from build123d import *

# Parameters (mm, degrees)
BOSS_EXTRUDE1_DEPTH    = 1.5
SKETCH2_W              = 30
SKETCH2_H              = 40
BOSS_EXTRUDE2_DEPTH    = 1.5
CONVERT_SOLID1_START   = -20
CONVERT_SOLID1_DEPTH   = 40
CONVERT_SOLID1_2_DEPTH = 40
M3_CLEARANCE_HOLE1_D   = 3.2
CIRPATTERN1_COUNT      = 6
CUT_EXTRUDE1_DEPTH     = 46.650848842
FILLET1_R              = 3
CUT_EXTRUDE2_DEPTH     = 1.5


# Read off the part's stored shape, not the designer's step: Convert-Solid1
with BuildPart() as part:
    # Sketch1 → Boss-Extrude1 (new body)
    with BuildSketch(Plane(origin=(0, 0, 0), x_dir=(0, 0, -1), z_dir=(1, 0, 0))):
        with BuildLine():
            Line((-20, 0), (-20, -28))
            Line((-20, -28), (20, -28))
            Line((20, -28), (20, 0))
            ThreePointArc((20, 0), (0, 20), (-20, 0))
        make_face()
    extrude(amount=BOSS_EXTRUDE1_DEPTH)

    # Sketch2 → Boss-Extrude2 (add)
    with BuildSketch(Plane.XZ.offset(28)):
        with Locations((15, 0)):
            Rectangle(SKETCH2_W, SKETCH2_H)
    extrude(amount=-BOSS_EXTRUDE2_DEPTH)

    # Convert-Solid1 outline → Convert-Solid1 (cut)
    with BuildSketch(Plane.XY.offset(CONVERT_SOLID1_START)):
        with BuildLine():
            Line((0, -28), (2.262, -28))
            ThreePointArc((2.262, -28), (0.662524461, -27.337475539), (0, -25.738))
            Line((0, -25.738), (0, -28))
        make_face()
    extrude(amount=CONVERT_SOLID1_DEPTH, mode=Mode.SUBTRACT)

    # Convert-Solid1 2 outline → Convert-Solid1 2 (add)
    with BuildSketch(Plane.XY.offset(CONVERT_SOLID1_START)):
        with BuildLine():
            Line((1.5, -26.5), (2.262, -26.5))
            ThreePointArc((2.262, -26.5), (1.723184633, -26.276815367), (1.5, -25.738))
            Line((1.5, -25.738), (1.5, -26.5))
        make_face()
    extrude(amount=CONVERT_SOLID1_2_DEPTH)

    # M3 Clearance Hole1 (through all)
    with Locations(Plane.ZY):
        with Locations((-15.5, 0)):
            m3_clearance_hole1 = Hole(M3_CLEARANCE_HOLE1_D / 2)

    # CirPattern1: M3 Clearance Hole1 ×6 about axis
    cirpattern1_axis = Axis((0, 0, 0), (1, 0, 0))
    for i in range(1, CIRPATTERN1_COUNT):
        add(m3_clearance_hole1.rotate(cirpattern1_axis, i * 360 / CIRPATTERN1_COUNT), mode=Mode.SUBTRACT)

    # Sketch9 → Cut-Extrude1 (cut, through all)
    with BuildSketch(Plane.ZY):
        with BuildLine():
            Line((6.25, 7), (6.25, -7))
            ThreePointArc((6.25, -7), (0, -13.25), (-6.25, -7))
            Line((-6.25, -7), (-6.25, 7))
            ThreePointArc((-6.25, 7), (0, 13.25), (6.25, 7))
        make_face()
    extrude(amount=-CUT_EXTRUDE1_DEPTH, mode=Mode.SUBTRACT)

    # Fillet1
    fillet1_edges = [part.edges().sort_by_distance(p)[0] for p in [
        (30, -27.25, 20),
        (30, -27.25, -20),
    ]]
    fillet(fillet1_edges, radius=FILLET1_R)

    # Sketch10 → Cut-Extrude2 (cut)
    with BuildSketch(Plane(origin=(0, -28, 0), x_dir=(-1, 0, 0), z_dir=(0, -1, 0))):
        with BuildLine():
            Line((-9.5, -16.65), (-23.5, -16.65))
            ThreePointArc((-23.5, -16.65), (-25.6, -14.55), (-23.5, -12.45))
            Line((-23.5, -12.45), (-9.5, -12.45))
            ThreePointArc((-9.5, -12.45), (-7.4, -14.55), (-9.5, -16.65))
        make_face()
        with BuildLine():
            Line((-7.4, 7), (-7.4, -7))
            ThreePointArc((-7.4, -7), (-9.5, -9.1), (-11.6, -7))
            Line((-11.6, -7), (-11.6, 7))
            ThreePointArc((-11.6, 7), (-9.5, 9.1), (-7.4, 7))
        make_face()
        with BuildLine():
            Line((-21.4, 7), (-21.4, -7))
            ThreePointArc((-21.4, -7), (-23.5, -9.1), (-25.6, -7))
            Line((-25.6, -7), (-25.6, 7))
            ThreePointArc((-25.6, 7), (-23.5, 9.1), (-21.4, 7))
        make_face()
        with BuildLine():
            Line((-9.5, 16.65), (-23.5, 16.65))
            ThreePointArc((-23.5, 16.65), (-25.6, 14.55), (-23.5, 12.45))
            Line((-23.5, 12.45), (-9.5, 12.45))
            ThreePointArc((-9.5, 12.45), (-7.4, 14.55), (-9.5, 16.65))
        make_face()
    extrude(amount=-CUT_EXTRUDE2_DEPTH, mode=Mode.SUBTRACT)


solid = part.part
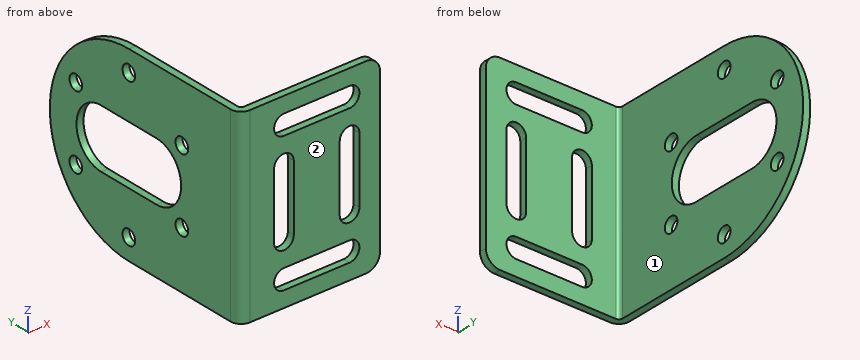
Design review of the part built by this model. Coordinates are the model's own, in mm. Face numbers are marked on the shaded views. A direction names the side the tool comes from. Coordinates: 2 decimals unless noted, no trailing zeros. Loops run counter-clockwise (first coordinate to the right, second up) from the corner with the lowest first, then second, coordinate; pieces in that order, holes last. Notation, with made-up numbers: (-35.75, -32) -> (-12.75, -32) arc R23 cw to (-12.75, 7) -> close; hole circle Ø5 at (30.25, 24.5). An arc over 180 degrees is marked (long way). Use a Markdown table: item, result. Add a question column.
Item 1: We need section B-B, the plane z = 0.5. Write out the cut boundary in (x, y), and give its area (3 significant figures).
Item 2: Clearance check with flat-ended pins moving along their axes: P1, Ø6, axis at y = 5.5, z = 8.5, coming from the +X side; P2, Ø1, axis at x = 14.5, z = 7.5, coming from the +Y side; P3, Ø0.8, axis at y = -27.5, z = 1, coming from the -X side. State where each tip first meets the part, or that it passes through.
Item 3: We need section D-D, the plane z = -15.5. Write out the cut boundary in (x, y), and give its area (3 significant figures).
Item 4: Wall thickness on L1, parallel to Y at x = 27.5, z = -17; L2, parallel to Y at x = 0.55, z = 7.75; L3, parallel to X at y = -9.5, z = -10: over which ranges is each line inside the solid? List them lowest first. Write a range as from..to.
Item 5: We need section C-C, the plane y = 1. Write out the cut boundary in (x, z), and give its area (3 significant figures).
Item 6: Machinability: for the marked faces 1 and 2, which of the approach directions +Z, -Z, +X, -X, +Y, -Y give a long, thin tool a straight path to every point of the face, cutting with its end or side? Answer none if there is none.
Item 7: We need section A-A, the plane x = 18.75. Write out the cut boundary in (y, z).
Numbers:
| question | item | result |
|---|---|---|
| 1 | outline | (0, -25.74) arc R2.26 ccw to (2.26, -28) -> (7.4, -28) -> (7.4, -26.5) -> (2.26, -26.5) arc R0.76 cw to (1.5, -25.74) -> (1.5, -13.23) -> (0, -13.23) -> close; (0, 13.23) -> (1.5, 13.23) -> (1.5, 19.99) -> (0, 19.99) -> close; (11.6, -28) -> (21.4, -28) -> (21.4, -26.5) -> (11.6, -26.5) -> close; (25.6, -28) -> (30, -28) -> (30, -26.5) -> (25.6, -26.5) -> close |
| 1 | area | 61.5 mm^2 |
| 2 | P1 | stops at x = 1.5 |
| 2 | P2 | stops at y = -26.5 |
| 2 | P3 | stops at x = 0.46 |
| 3 | outline | (0, -25.74) arc R2.26 ccw to (2.26, -28) -> (7.63, -28) -> (7.63, -26.5) -> (2.26, -26.5) arc R0.76 cw to (1.5, -25.74) -> (1.5, -1.6) -> (0, -1.6) -> close; (0, 1.6) -> (1.5, 1.6) -> (1.5, 12.64) -> (0, 12.64) -> close; (25.37, -28) -> (30, -28) -> (30, -26.5) -> (25.37, -26.5) -> close |
| 3 | area | 71.3 mm^2 |
| 4 | L1 | y = -28..-26.5 |
| 4 | L2 | y = -27.22..-15.02, -11.82..11.82, 15.02..18.44 |
| 4 | L3 | x = 0..1.5 |
| 5 | outline | (0, -19.97) -> (1.5, -19.97) -> (1.5, -16.75) -> (0, -16.75) -> close; (0, -14.25) -> (1.5, -14.25) -> (1.5, -6.25) -> (0, -6.25) -> close; (0, 6.25) -> (1.5, 6.25) -> (1.5, 14.25) -> (0, 14.25) -> close; (0, 16.75) -> (1.5, 16.75) -> (1.5, 19.97) -> (0, 19.97) -> close |
| 5 | area | 33.7 mm^2 |
| 6 | face 1 | +Z, -Z, +X, +Y |
| 6 | face 2 | +Z, -Z, +X, -X, -Y |
| 7 | outline | (-28, -20) -> (-26.5, -20) -> (-26.5, -16.65) -> (-28, -16.65) -> close; (-28, -12.45) -> (-26.5, -12.45) -> (-26.5, 12.45) -> (-28, 12.45) -> close; (-28, 16.65) -> (-26.5, 16.65) -> (-26.5, 20) -> (-28, 20) -> close |
